Geometry: final body of the model. Coordinates: model frame, mm. Round coordinates to 2 decimals unless told otherwise and drop trailing zeros. Write each loop counter-clockwise with the first axis right and the second up, starting at its lowest first coordinate (ties: lowest second). Pieces come first, ordered by that corner, then holes. Notation, with made-up numbers: M 38,82.5 L 86,82.5 A23 ccw 86,100.5 Z; hole C -19,30 d10. An arc over 180 degrees is marked long. Use one line per item in the form item = value. Start each with the question number.
Item 1: Section query C-C (y = -2.5). Return loops of the section in (x, z), and give its area (3 significant figures).
Item 2: Section query A-A (x = 0). Return loops of the section in (y, z), and give its area (3 significant figures).
Item 3: Pin query (flat end, axial travel): pin 1 Ø2 at (y, z) = (158.5, -54.5) entering from -X; pin 2 Ø3 at (y, z) = (58, -10) entering from -X; pin 3 Ø1.5 at (y, z) = (18.5, -4.5) entering from -X. Return the tip coordinate at first contact, or that it passes through.
Item 4: Ray query, probe 1 along X at (y, z) = (91.5, 0); probe 2 along Z at (x, y) = (1, 145.5); probe 3 along Z at (x, y) = (11, 68.5). Return the intervals inside material, ascending.
Item 5: Section query B-B (z = 0). Return loops of the section in (x, y), and give its area (3 significant figures).
Item 6: Section query D-D (y = 22.5). Return loops of the section in (x, z), and give its area (3 significant figures).
from build123d import *
from build123d.topology import SkipClean

# Parameters (mm, degrees)
SKETCH1_R           = 57.15
SKETCH1_R_2         = 54.61
BOSS_EXTRUDE1_DEPTH = 152.4
BOSS_EXTRUDE2_DEPTH = 15.24
BOSS_EXTRUDE3_START = 15.24
BOSS_EXTRUDE3_DEPTH = 15.24


with BuildPart() as part:
    # Sketch1 → Boss-Extrude1 (new body)
    with BuildSketch(Plane(origin=(0, 0, 0), x_dir=(1, 0, 0), z_dir=(0, 1, 0))):
        with Locations(Location((0, 0, 0), (0, 0, 90))):
            Circle(SKETCH1_R)
        with Locations(Location((0, 0, 0), (0, 0, 90))):
            Circle(SKETCH1_R_2, mode=Mode.SUBTRACT)
    extrude(amount=BOSS_EXTRUDE1_DEPTH)

    # Sketch2 → Boss-Extrude2 (add)
    with SkipClean():  # the faces are left unmerged after this step: merging them gives an invalid solid
        with BuildSketch(Plane(origin=(0, 152.4, 0), x_dir=(1, 0, 0), z_dir=(0, 1, 0))):
            with BuildLine():
                Line((-55.99533552, 11.43), (-53.400441946, 11.43))
                ThreePointArc((-53.400441946, 11.43), (-54.61, 0), (-53.400441946, -11.43))
                Line((-53.400441946, -11.43), (-55.99533552, -11.43))
                ThreePointArc((-55.99533552, -11.43), (-57.15, 0), (-55.99533552, 11.43))
            make_face()
            with BuildLine():
                Line((11.43, 53.400441946), (11.43, 55.99533552))
                ThreePointArc((11.43, 55.99533552), (0, 57.15), (-11.43, 55.99533552))
                Line((-11.43, 55.99533552), (-11.43, 53.400441946))
                ThreePointArc((-11.43, 53.400441946), (0, 54.61), (11.43, 53.400441946))
            make_face()
            with BuildLine():
                Line((53.400441946, 11.43), (55.99533552, 11.43))
                ThreePointArc((55.99533552, 11.43), (57.15, 0), (55.99533552, -11.43))
                Line((55.99533552, -11.43), (53.400441946, -11.43))
                ThreePointArc((53.400441946, -11.43), (54.61, 0), (53.400441946, 11.43))
            make_face()
            with BuildLine():
                Line((-11.43, -53.400441946), (-11.43, -55.99533552))
                ThreePointArc((-11.43, -55.99533552), (-0.008316105, -57.149999395), (11.413703346, -55.998659591))
                Line((11.413703346, -55.998659591), (11.43, -53.400441946))
                ThreePointArc((11.43, -53.400441946), (0, -54.61), (-11.43, -53.400441946))
            make_face()
        extrude(amount=BOSS_EXTRUDE2_DEPTH)

    # Sketch3 → Boss-Extrude3 (add)
    with SkipClean():  # the faces are left unmerged after this step: merging them gives an invalid solid
        with BuildSketch(Plane.XZ.offset(BOSS_EXTRUDE3_START)):
            with BuildLine():
                Line((11.43, 55.99533552), (11.43, 53.400441946))
                ThreePointArc((11.43, 53.400441946), (0, 54.61), (-11.43, 53.400441946))
                Line((-11.43, 53.400441946), (-11.43, 55.99533552))
                ThreePointArc((-11.43, 55.99533552), (0, 57.15), (11.43, 55.99533552))
            make_face()
            with BuildLine():
                Line((53.400441946, 11.43), (55.99533552, 11.43))
                ThreePointArc((55.99533552, 11.43), (57.15, 0), (55.99533552, -11.43))
                Line((55.99533552, -11.43), (53.400441946, -11.43))
                ThreePointArc((53.400441946, -11.43), (54.61, 0), (53.400441946, 11.43))
            make_face()
            with BuildLine():
                Line((-11.43, -53.400441946), (-11.43, -55.99533552))
                ThreePointArc((-11.43, -55.99533552), (0, -57.15), (11.43, -55.99533552))
                Line((11.43, -55.99533552), (11.43, -53.400441946))
                ThreePointArc((11.43, -53.400441946), (0, -54.61), (-11.43, -53.400441946))
            make_face()
            with BuildLine():
                Line((-55.99533552, 11.43), (-53.400441946, 11.43))
                ThreePointArc((-53.400441946, 11.43), (-54.61, 0), (-53.400441946, -11.43))
                Line((-53.400441946, -11.43), (-55.99533552, -11.43))
                ThreePointArc((-55.99533552, -11.43), (-57.15, 0), (-55.99533552, 11.43))
            make_face()
        extrude(amount=-BOSS_EXTRUDE3_DEPTH)


solid = part.part
Working result:
q1.outline = M -56,-11.43 L -53.4,-11.43 A54.61 cw -53.4,11.43 L -56,11.43 A57.15 ccw Z; M -11.43,-56 A57.15 ccw 11.43,-56 L 11.43,-53.4 A54.61 cw -11.43,-53.4 Z; M -11.43,53.4 A54.61 cw 11.43,53.4 L 11.43,56 A57.15 ccw -11.43,56 Z; M 53.4,-11.43 L 56,-11.43 A57.15 ccw 56,11.43 L 53.4,11.43 A54.61 cw Z
q1.area = 234 mm²
q2.outline = M -15.24,-57.15 L 167.64,-57.15 L 167.64,-54.61 L -15.24,-54.61 Z; M -15.24,54.61 L 167.64,54.61 L 167.64,57.15 L -15.24,57.15 Z
q2.area = 929 mm²
q3.pin_1 = -11.43
q3.pin_2 = -56.51
q3.pin_3 = -57.03
q4.probe_1 = -57.15 to -54.61, 54.61 to 57.15
q4.probe_2 = -57.14 to -54.6, 54.6 to 57.14
q4.probe_3 = -56.08 to -53.49, 53.49 to 56.08
q5.outline = M -57.15,-15.24 L -54.61,-15.24 L -54.61,167.64 L -57.15,167.64 Z; M 54.61,-15.24 L 57.15,-15.24 L 57.15,167.64 L 54.61,167.64 Z
q5.area = 929 mm²
q6.outline = C 0,0 d114.3; hole C 0,0 d109.22
q6.area = 892 mm²
